```python
from build123d import *

# Parameters (mm, degrees)
SKETCH1_W           = 11.9
SKETCH1_H           = 5.95
BOSS_EXTRUDE1_DEPTH = 250
CUT_EXTRUDE1_DEPTH  = 251


with BuildPart() as part:
    # Sketch1 → Boss-Extrude1 (new body)
    with BuildSketch(Plane.XY):
        with BuildLine():
            Line((-4.350229073, 14.992640687), (-13.192640687, 14.992640687))
            ThreePointArc((-13.192640687, 14.992640687), (-14.465432893, 14.465432893), (-14.992640687, 13.192640687))
            Line((-14.992640687, 13.192640687), (-14.992640687, 4.350229073))
            Line((-14.992640687, 4.350229073), (-13.792640687, 4.350229073))
            ThreePointArc((-13.792640687, 4.350229073), (-13.085533906, 4.643122292), (-12.792640687, 5.350229073))
            Line((-12.792640687, 5.350229073), (-12.792640687, 8.460229073))
            Line((-12.792640687, 8.460229073), (-8.460229073, 8.460229073))
            Line((-8.460229073, 8.460229073), (-8.460229073, 12.792640687))
            Line((-8.460229073, 12.792640687), (-5.350229073, 12.792640687))
            ThreePointArc((-5.350229073, 12.792640687), (-4.643122292, 13.085533906), (-4.350229073, 13.792640687))
            Line((-4.350229073, 13.792640687), (-4.350229073, 14.992640687))
        make_face()
        with BuildLine():
            Line((-10.660229073, 13.792640687), (-12.792640687, 13.792640687))
            ThreePointArc((-12.792640687, 13.792640687), (-13.499747468, 13.499747468), (-13.792640687, 12.792640687))
            Line((-13.792640687, 12.792640687), (-13.792640687, 10.660229073))
            ThreePointArc((-13.792640687, 10.660229073), (-13.499747468, 9.953122292), (-12.792640687, 9.660229073))
            Line((-12.792640687, 9.660229073), (-10.660229073, 9.660229073))
            ThreePointArc((-10.660229073, 9.660229073), (-9.953122292, 9.953122292), (-9.660229073, 10.660229073))
            Line((-9.660229073, 10.660229073), (-9.660229073, 12.792640687))
            ThreePointArc((-9.660229073, 12.792640687), (-9.953122292, 13.499747468), (-10.660229073, 13.792640687))
        make_face(mode=Mode.SUBTRACT)
        Polygon((-5.95, 4.217588386), (-5.95, 5.95), (-4.217588386, 5.95), (-8.460229073, 10.192640687), (-8.460229073, 8.460229073), (-10.192640687, 8.460229073), align=None)
        with Locations((0, 2.975)):
            Rectangle(SKETCH1_W, SKETCH1_H)
        Polygon((8.460229073, 10.192640687), (4.217588386, 5.95), (5.95, 5.95), (5.95, 4.217588386), (10.192640687, 8.460229073), (8.460229073, 8.460229073), align=None)
        with BuildLine():
            Line((12.792640687, 8.460229073), (12.792640687, 5.350229073))
            ThreePointArc((12.792640687, 5.350229073), (13.085533906, 4.643122292), (13.792640687, 4.350229073))
            Line((13.792640687, 4.350229073), (14.992640687, 4.350229073))
            Line((14.992640687, 4.350229073), (14.992640687, 13.192640687))
            ThreePointArc((14.992640687, 13.192640687), (14.465432893, 14.465432893), (13.192640687, 14.992640687))
            Line((13.192640687, 14.992640687), (4.350229073, 14.992640687))
            Line((4.350229073, 14.992640687), (4.350229073, 13.792640687))
            ThreePointArc((4.350229073, 13.792640687), (4.643122292, 13.085533906), (5.350229073, 12.792640687))
            Line((5.350229073, 12.792640687), (8.460229073, 12.792640687))
            Line((8.460229073, 12.792640687), (8.460229073, 8.460229073))
            Line((8.460229073, 8.460229073), (12.792640687, 8.460229073))
        make_face()
        with BuildLine():
            ThreePointArc((9.660229073, 10.660229073), (9.953122292, 9.953122292), (10.660229073, 9.660229073))
            Line((10.660229073, 9.660229073), (12.792640687, 9.660229073))
            ThreePointArc((12.792640687, 9.660229073), (13.499747468, 9.953122292), (13.792640687, 10.660229073))
            Line((13.792640687, 10.660229073), (13.792640687, 12.792640687))
            ThreePointArc((13.792640687, 12.792640687), (13.499747468, 13.499747468), (12.792640687, 13.792640687))
            Line((12.792640687, 13.792640687), (10.660229073, 13.792640687))
            ThreePointArc((10.660229073, 13.792640687), (9.953122292, 13.499747468), (9.660229073, 12.792640687))
            Line((9.660229073, 12.792640687), (9.660229073, 10.660229073))
        make_face(mode=Mode.SUBTRACT)
    extrude(amount=-BOSS_EXTRUDE1_DEPTH)

    # Mirror1: part across plane


with BuildPart() as part_1:
    add(part.part)
    add(part.part.mirror(Plane(origin=(0, 0, -250), x_dir=(0, 0, 1), z_dir=(0, -1, 0))))

    # Sketch2 → Cut-Extrude1 (cut, through all)
    with BuildSketch(Plane.XY):
        with BuildLine():
            Line((-4.631549417, 3.075914498), (-3.16821753, 1.612582612))
            ThreePointArc((-3.16821753, 1.612582612), (-2.513764607, 2.513764607), (-1.612582612, 3.16821753))
            Line((-1.612582612, 3.16821753), (-3.075914498, 4.631549417))
            Line((-3.075914498, 4.631549417), (-4.631549417, 3.075914498))
        make_face()
        with BuildLine():
            Line((-3.16821753, 1.612582612), (-1.555634919, 0))
            Line((-1.555634919, 0), (0, 1.555634919))
            Line((0, 1.555634919), (-1.612582612, 3.16821753))
            ThreePointArc((-1.612582612, 3.16821753), (-2.513764607, 2.513764607), (-3.16821753, 1.612582612))
        make_face()
        with BuildLine():
            ThreePointArc((-3.16821753, 1.612582612), (-3.555, 0), (-3.16821753, -1.612582612))
            Line((-3.16821753, -1.612582612), (-1.555634919, 0))
            Line((-1.555634919, 0), (-3.16821753, 1.612582612))
        make_face()
        with BuildLine():
            Line((-4.631549417, -3.075914498), (-3.075914498, -4.631549417))
            Line((-3.075914498, -4.631549417), (-1.612582612, -3.16821753))
            ThreePointArc((-1.612582612, -3.16821753), (-2.513764607, -2.513764607), (-3.16821753, -1.612582612))
            Line((-3.16821753, -1.612582612), (-4.631549417, -3.075914498))
        make_face()
        with BuildLine():
            ThreePointArc((-3.16821753, -1.612582612), (-2.513764607, -2.513764607), (-1.612582612, -3.16821753))
            Line((-1.612582612, -3.16821753), (0, -1.555634919))
            Line((0, -1.555634919), (-1.555634919, 0))
            Line((-1.555634919, 0), (-3.16821753, -1.612582612))
        make_face()
        with BuildLine():
            Line((0, -1.555634919), (-1.612582612, -3.16821753))
            ThreePointArc((-1.612582612, -3.16821753), (0, -3.555), (1.612582612, -3.16821753))
            Line((1.612582612, -3.16821753), (0, -1.555634919))
        make_face()
        with BuildLine():
            Line((1.555634919, 0), (0, -1.555634919))
            Line((0, -1.555634919), (1.612582612, -3.16821753))
            ThreePointArc((1.612582612, -3.16821753), (2.513764607, -2.513764607), (3.16821753, -1.612582612))
            Line((3.16821753, -1.612582612), (1.555634919, 0))
        make_face()
        with BuildLine():
            Line((3.16821753, 1.612582612), (1.555634919, 0))
            Line((1.555634919, 0), (3.16821753, -1.612582612))
            ThreePointArc((3.16821753, -1.612582612), (3.456952294, -0.829159719), (3.555, 0))
            ThreePointArc((3.555, 0), (3.456952294, 0.829159719), (3.16821753, 1.612582612))
        make_face()
        Polygon((-1.555634919, 0), (0, -1.555634919), (1.555634919, 0), (0, 1.555634919), align=None)
        with BuildLine():
            Line((0, 1.555634919), (1.555634919, 0))
            Line((1.555634919, 0), (3.16821753, 1.612582612))
            ThreePointArc((3.16821753, 1.612582612), (2.513764607, 2.513764607), (1.612582612, 3.16821753))
            Line((1.612582612, 3.16821753), (0, 1.555634919))
        make_face()
        with BuildLine():
            Line((-1.612582612, 3.16821753), (0, 1.555634919))
            Line((0, 1.555634919), (1.612582612, 3.16821753))
            ThreePointArc((1.612582612, 3.16821753), (0, 3.555), (-1.612582612, 3.16821753))
        make_face()
        with BuildLine():
            ThreePointArc((1.612582612, 3.16821753), (2.513764607, 2.513764607), (3.16821753, 1.612582612))
            Line((3.16821753, 1.612582612), (4.631549417, 3.075914498))
            Line((4.631549417, 3.075914498), (3.075914498, 4.631549417))
            Line((3.075914498, 4.631549417), (1.612582612, 3.16821753))
        make_face()
        with BuildLine():
            ThreePointArc((3.16821753, -1.612582612), (2.513764607, -2.513764607), (1.612582612, -3.16821753))
            Line((1.612582612, -3.16821753), (3.075914498, -4.631549417))
            Line((3.075914498, -4.631549417), (4.631549417, -3.075914498))
            Line((4.631549417, -3.075914498), (3.16821753, -1.612582612))
        make_face()
    extrude(amount=-CUT_EXTRUDE1_DEPTH, mode=Mode.SUBTRACT)


solid = part_1.part
```
For this review, take the finished solid that the model builds, in its own axes (mm). A direction names the side the tool comes from. Give positions to 0.01 mm unless a question says otherwise; leave off trailing zeros.
Item 1: Wall thickness on probe 1 along X at (y, z) = (-11, -29); probe 2 along X at (y, z) = (5.25, -118.5): over which ranges is each line inside the solid? List them lowest first.
Item 2: Machinability: for faces 5 (the face through (6.37, 8.1, -123.25)), 6 (the face through (5.95, 0, -123)), 7 (the face through (0, -5.95, -123)), 8 (the face through (0, 5.95, -123)), which of the approach directions +Z, -Z, +X, -X, +Y, -Y give a long, thin tool a straight path to every point of the face, cutting with its end or side? Answer none if there is none.
Item 3: Insertion check: P1, Ø4, axis at y = 1.5, z = -185.5, coming from the +X side; P2, Ø1.3, axis at y = 14.5, z = -169.5, coming from the +X side; P3, Ø1, axis at y = 14.5, z = -106.5, coming from the -X side. Each pin has a flat end and moves straight along its axis. Give the tip position at first contact, or say it passes through.
Item 4: The part is to be moulded in two halves that separate along Y. For faces 1 (the face through (8.04, -6.31, -123.25)), 2 (the face through (9, -14.993, -123)), 3 (the face through (6.37, -8.1, -123.25)), 4 (the face through (9, 14.993, -123)), say which applies: +Y half, -Y half, draft (parallel to the pull), parting line (faces both ways), or undercut.
Item 5: Take a section at A-A (z = -220.5). Give the number of separate pieces and of enclosed holes in the cut face, and give its area (3 significant figures).
Established:
1. probe 1: x = -14.99 to -13.79, -9.66 to -8.46, 8.46 to 9.66, 13.79 to 14.99
1. probe 2: x = -14.99 to -12.8, -6.98 to 6.98, 12.8 to 14.99
2. face 5: +Z, -Z
2. face 6: +Z, -Z, +X
2. face 7: +Z, -Z, -Y
2. face 8: +Z, -Z, +Y
3. P1: stops at x = 5.95
3. P2: stops at x = 14.87
3. P3: stops at x = -14.8
4. face 1: undercut
4. face 2: -Y half
4. face 3: undercut
4. face 4: +Y half
5. separate pieces: 1
5. enclosed holes: 5
5. area: 305 mm2
